Read the model definition and answer for the solid it produces. Units are mm, in the model's axes. A direction names the side the tool comes from. Give positions to 0.01 mm unless a question says otherwise; leave off trailing zeros. Loops run counter-clockwise (first coordinate to the right, second up) from the corner with the lowest first, then second, coordinate; pieces in that order, holes last.
(1) Each of these flat-tipped pins is pushed along its axis until it touches: P1, Ø3, axis at y = 15, z = -7, coming from the -X side; P2, Ø8, axis at x = -20, z = 0, coming from the +Y side; P3, Ø4.5, axis at x = 20, z = 0, coming from the +Y side. Where does it stop, or does it pass through?
(2) Straight lines are drawn through the part: probe 1 along X at (y, z) = (49.05, 0); probe 2 along X at (y, z) = (49.65, 20); probe 3 along Y at (x, z) = (-0.5, -15.5). For each, find the intervals that lie inside material, in ascending order.
(3) Determine the mould class of faces 1 (the face through (2, 65, 5)), 2 (the face through (22.48, 49.26, -0.33)), 3 (the face through (8.396, 62.395, -2.644)) for opening direction X: pulls with the +X half, pulls with the -X half, needs draft (parallel to the pull), parting line crosses it, or undercut.
(4) Find section A-A, the plane x = 0. Write down the section's boundary in (y, z).
(5) Find section C-C, the plane y = 22.5. Write down the section's boundary in (x, z), then the cut area to 3 significant figures.
(6) Find section D-D, the plane x = 20. Write down the section's boundary in (y, z).
(7) Which of the six approach directions +Z, -Z, +X, -X, +Y, -Y give full straight-line access (tool end or side, diameter ignored) to faces 4 (the face through (-17.52, 49.26, -0.33)), 5 (the face through (7.509, 24.65, 23.846))?
(8) Find section B-B, the plane z = -20. Write down the section's boundary in (x, y), then the cut area to 3 significant figures.
```python
from build123d import *

# Parameters (mm, degrees)
SKETCH1_R           = 25
BOSS_EXTRUDE1_DEPTH = 50
SKETCH3_R           = 7.5
SKETCH4_R           = 15
SKETCH5_R           = 5
CUT_EXTRUDE1_DEPTH  = 0.5
CUT_EXTRUDE2_START  = -15
SKETCH5_4_R         = 2.5
CUT_EXTRUDE2_DEPTH  = 1.5


with BuildPart() as part:
    # Sketch1 → Boss-Extrude1 (new body)
    with BuildSketch(Plane(origin=(0, 0, 0), x_dir=(1, 0, 0), z_dir=(0, 1, 0))):
        with Locations(Location((0, 0, 0), (0, 0, 270))):
            Circle(SKETCH1_R)
    extrude(amount=BOSS_EXTRUDE1_DEPTH)

    # Sketch3 → Loft1 section 0
    with BuildSketch(Plane(origin=(0, 65, 0), x_dir=(1, 0, 0), z_dir=(0, 1, 0))):
        Circle(SKETCH3_R)
    # Sketch4 → Loft1 section 1
    with BuildSketch(Plane(origin=(0, 50, 0), x_dir=(1, 0, 0), z_dir=(0, 1, 0))):
        Circle(SKETCH4_R)
    loft()

    # Sketch5 → Cut-Extrude1 (cut)
    with BuildSketch(Plane(origin=(0, 65, 0), x_dir=(1, 0, 0), z_dir=(0, 1, 0))):
        with Locations(Location((0, 0, 0), (0, 0, 270))):
            Circle(SKETCH5_R)
    extrude(amount=-CUT_EXTRUDE1_DEPTH, mode=Mode.SUBTRACT)

    # Sketch5<4> → Cut-Extrude2 (cut)
    with BuildSketch(Plane(origin=(0, 65, 0), x_dir=(1, 0, 0), z_dir=(0, 1, 0)).offset(CUT_EXTRUDE2_START)):
        with Locations(Location((-20, 0, 0), (0, 0, 270))):
            Circle(SKETCH5_4_R)
        with Locations(Location((0, 20, 0), (0, 0, 270))):
            Circle(SKETCH5_4_R)
        with Locations(Location((20, 0, 0), (0, 0, 270))):
            Circle(SKETCH5_4_R)
        with Locations(Location((0, -20, 0), (0, 0, 270))):
            Circle(SKETCH5_4_R)
    extrude(amount=-CUT_EXTRUDE2_DEPTH, mode=Mode.SUBTRACT)


solid = part.part
```
Entries:
1. P1: stops at x = -24.39
1. P2: stops at y = 50
1. P3: stops at y = 48.5
2. probe 1: x = -25 to -22.5, -17.5 to 17.5, 22.5 to 25
2. probe 2: x = -15 to -2.5, 2.5 to 15
2. probe 3: y = 0 to 50
3. face 1: needs draft
3. face 2: undercut
3. face 3: parting line crosses it
4. outline: (0, -25) - (50, -25) - (50, -22.5) - (48.5, -22.5) - (48.5, -17.5) - (50, -17.5) - (50, -15) - (65, -7.5) - (65, -5) - (64.5, -5) - (64.5, 5) - (65, 5) - (65, 7.5) - (50, 15) - (50, 17.5) - (48.5, 17.5) - (48.5, 22.5) - (50, 22.5) - (50, 25) - (0, 25) - close
5. outline: circle Ø50 at (0, 0)
5. area: 1,960 mm2
6. outline: (0, -15) - (50, -15) - (50, -2.5) - (48.5, -2.5) - (48.5, 2.5) - (50, 2.5) - (50, 15) - (0, 15) - close
7. face 4: +Y
7. face 5: +Y, -Y
8. outline: (-15, 0) - (15, 0) - (15, 50) - (2.5, 50) - (2.5, 48.5) - (-2.5, 48.5) - (-2.5, 50) - (-15, 50) - close
8. area: 1,490 mm2
